from build123d import *

# Parameters (mm, degrees)
EXTRUDE_1_DEPTH             = 90
SKETCH_2_W                  = 90
SKETCH_2_H                  = 44.25
EXTRUDE_2_DEPTH             = 8.2
SKETCH_3_W                  = 90
SKETCH_3_H                  = 102.45
EXTRUDE_3_DEPTH             = 8.2
SKETCH_4_W                  = 4.5
SKETCH_4_H                  = 3.95
CUT_EXTRUDE_1_DEPTH         = 91
SKETCH_5_W                  = 2.25
SKETCH_5_H                  = 3.95
CUT_EXTRUDE_2_DEPTH         = 91
SKETCH_6_W                  = 3.95
SKETCH_6_H                  = 2.25
CUT_EXTRUDE_3_DEPTH         = 91
SKETCH_7_W                  = 3.95
SKETCH_7_H                  = 29.5
CUT_EXTRUDE_4_DEPTH         = 91
SKETCH_8_W                  = 3.95
SKETCH_8_H                  = 9
CUT_EXTRUDE_5_DEPTH         = 91
SKETCH_9_W                  = 3.95
SKETCH_9_H                  = 29.5
CUT_EXTRUDE_6_DEPTH         = 91
SKETCH_10_W                 = 3.95
SKETCH_10_H                 = 6.2
CUT_EXTRUDE_7_DEPTH         = 91
SKETCH_11_W                 = 2.25
SKETCH_11_H                 = 3.95
CUT_EXTRUDE_8_DEPTH         = 91
SKETCH_12_W                 = 4.5
SKETCH_12_H                 = 3.95
CUT_EXTRUDE_9_DEPTH         = 91
SKETCH_13_W                 = 9
SKETCH_13_H                 = 3.95
CUT_EXTRUDE_10_DEPTH        = 91
SKETCH_14_W                 = 46.1
SKETCH_14_H                 = 96.1
CUT_EXTRUDE_11_DEPTH        = 86.6
HOLE_WIZARD_2_5_2_5_1_D     = 2.5
HOLE_WIZARD_2_5_2_5_1_DEPTH = 90
HOLE_WIZARD_4_5_4_5_1_D     = 4.5
HOLE_WIZARD_4_5_4_5_1_DEPTH = 90
SKETCH_22_R                 = 1.631577579
SKETCH_22_R_2               = 1.519375383
SKETCH_22_R_3               = 1.487580747
SKETCH_22_R_4               = 1.581735942
SKETCH_22_R_5               = 1.487835557
SKETCH_22_R_6               = 1.42600834
SKETCH_22_R_7               = 1.628129915
SKETCH_22_R_8               = 1.52367125
EXTRUDE_4_DEPTH             = 90
FILLET_5_R                  = 2
FILLET_6_R                  = 2
FILLET_7_R                  = 2
FILLET_8_R                  = 2
FILLET_9_R                  = 2
FILLET_10_R                 = 2
FILLET_11_R                 = 2
FILLET_12_R                 = 2
FILLET_13_R                 = 2
FILLET_14_R                 = 2
FILLET_15_R                 = 2
FILLET_16_R                 = 2
FILLET_17_R                 = 2
FILLET_18_R                 = 2
FILLET_19_R                 = 2
FILLET_20_R                 = 2
EXTRUDE_6_DEPTH             = 0.2


with BuildPart() as part:
    # Эскиз1 → Бобышка-Вытянуть1 (new body)
    with BuildSketch(Plane(origin=(90, 0, 0), x_dir=(0, 0, -1), z_dir=(1, 0, 0))):
        with BuildLine():
            Line((6.75, 225.906238208), (6.75, 320.75))
            Line((6.75, 320.75), (-38.093761792, 320.75))
            ThreePointArc((-38.093761792, 320.75), (-41.825, 319.5), (-38.093761792, 318.25))
            Line((-38.093761792, 318.25), (-37.5, 318.25))
            Line((-37.5, 318.25), (-37.5, 284.75))
            Line((-37.5, 284.75), (-38.093761792, 284.75))
            ThreePointArc((-38.093761792, 284.75), (-41.825, 283.5), (-38.093761792, 282.25))
            Line((-38.093761792, 282.25), (-37.5, 282.25))
            Line((-37.5, 282.25), (-37.5, 269.25))
            Line((-37.5, 269.25), (-38.093761792, 269.25))
            ThreePointArc((-38.093761792, 269.25), (-41.825, 268), (-38.093761792, 266.75))
            Line((-38.093761792, 266.75), (-37.5, 266.75))
            Line((-37.5, 266.75), (-37.5, 233.25))
            Line((-37.5, 233.25), (-38.093761792, 233.25))
            ThreePointArc((-38.093761792, 233.25), (-41.825, 232), (-38.093761792, 230.75))
            Line((-38.093761792, 230.75), (-37.5, 230.75))
            Line((-37.5, 230.75), (-37.5, 226.5))
            Line((-37.5, 226.5), (-33.25, 226.5))
            Line((-33.25, 226.5), (-33.25, 225.906238208))
            ThreePointArc((-33.25, 225.906238208), (-32, 222.175), (-30.75, 225.906238208))
            Line((-30.75, 225.906238208), (-30.75, 226.5))
            Line((-30.75, 226.5), (-22.25, 226.5))
            Line((-22.25, 226.5), (-22.25, 225.906238208))
            ThreePointArc((-22.25, 225.906238208), (-21, 222.175), (-19.75, 225.906238208))
            Line((-19.75, 225.906238208), (-19.75, 226.5))
            Line((-19.75, 226.5), (-6.75, 226.5))
            Line((-6.75, 226.5), (-6.75, 225.906238208))
            ThreePointArc((-6.75, 225.906238208), (-5.5, 222.175), (-4.25, 225.906238208))
            Line((-4.25, 225.906238208), (-4.25, 226.5))
            Line((-4.25, 226.5), (4.25, 226.5))
            Line((4.25, 226.5), (4.25, 225.906238208))
            ThreePointArc((4.25, 225.906238208), (5.5, 222.175), (6.75, 225.906238208))
        make_face()
    extrude(amount=-EXTRUDE_1_DEPTH)

    # Эскиз2 → Бобышка-Вытянуть2 (add)
    with BuildSketch(Plane(origin=(0, 320.75, 0), x_dir=(-1, 0, 0), z_dir=(0, 1, 0))):
        with Locations((-45, 15.375)):
            Rectangle(SKETCH_2_W, SKETCH_2_H)
    extrude(amount=EXTRUDE_2_DEPTH)

    # Эскиз3 → Бобышка-Вытянуть3 (add)
    with BuildSketch(Plane(origin=(0, 0, -6.75), x_dir=(-1, 0, 0), z_dir=(0, 0, -1))):
        with Locations((-45, 277.725)):
            Rectangle(SKETCH_3_W, SKETCH_3_H)
    extrude(amount=EXTRUDE_3_DEPTH)

    # Эскиз4 → Вырез-Вытянуть1 (cut, through all)
    with BuildSketch(Plane.ZY):
        with Locations((26.5, 326.975)):
            Rectangle(SKETCH_4_W, SKETCH_4_H)
    extrude(amount=-CUT_EXTRUDE_1_DEPTH, mode=Mode.SUBTRACT)

    # Эскиз5 → Вырез-Вытянуть2 (cut, through all)
    with BuildSketch(Plane.ZY):
        with Locations((36.375, 326.975)):
            Rectangle(SKETCH_5_W, SKETCH_5_H)
    extrude(amount=-CUT_EXTRUDE_2_DEPTH, mode=Mode.SUBTRACT)

    # Эскиз6 → Вырез-Вытянуть3 (cut, through all)
    with BuildSketch(Plane.ZY):
        with Locations((-12.975, 227.625)):
            Rectangle(SKETCH_6_W, SKETCH_6_H)
    extrude(amount=-CUT_EXTRUDE_3_DEPTH, mode=Mode.SUBTRACT)

    # Эскиз7 → Вырез-Вытянуть4 (cut, through all)
    with BuildSketch(Plane.ZY):
        with Locations((-12.975, 250)):
            Rectangle(SKETCH_7_W, SKETCH_7_H)
    extrude(amount=-CUT_EXTRUDE_4_DEPTH, mode=Mode.SUBTRACT)

    # Эскиз8 → Вырез-Вытянуть5 (cut, through all)
    with BuildSketch(Plane.ZY):
        with Locations((-12.975, 275.75)):
            Rectangle(SKETCH_8_W, SKETCH_8_H)
    extrude(amount=-CUT_EXTRUDE_5_DEPTH, mode=Mode.SUBTRACT)

    # Эскиз9 → Вырез-Вытянуть6 (cut, through all)
    with BuildSketch(Plane.ZY):
        with Locations((-12.975, 301.5)):
            Rectangle(SKETCH_9_W, SKETCH_9_H)
    extrude(amount=-CUT_EXTRUDE_6_DEPTH, mode=Mode.SUBTRACT)

    # Эскиз10 → Вырез-Вытянуть7 (cut, through all)
    with BuildSketch(Plane.ZY):
        with Locations((-12.975, 325.85)):
            Rectangle(SKETCH_10_W, SKETCH_10_H)
    extrude(amount=-CUT_EXTRUDE_7_DEPTH, mode=Mode.SUBTRACT)

    # Эскиз11 → Вырез-Вытянуть8 (cut, through all)
    with BuildSketch(Plane.ZY):
        with Locations((-9.875, 326.975)):
            Rectangle(SKETCH_11_W, SKETCH_11_H)
    extrude(amount=-CUT_EXTRUDE_8_DEPTH, mode=Mode.SUBTRACT)

    # Эскиз12 → Вырез-Вытянуть9 (cut, through all)
    with BuildSketch(Plane.ZY):
        with Locations((0, 326.975)):
            Rectangle(SKETCH_12_W, SKETCH_12_H)
    extrude(amount=-CUT_EXTRUDE_9_DEPTH, mode=Mode.SUBTRACT)

    # Эскиз13 → Вырез-Вытянуть10 (cut, through all)
    with BuildSketch(Plane.ZY):
        with Locations((13.25, 326.975)):
            Rectangle(SKETCH_13_W, SKETCH_13_H)
    extrude(amount=-CUT_EXTRUDE_10_DEPTH, mode=Mode.SUBTRACT)

    # Эскиз14 → Вырез-Вытянуть11 (cut)
    with BuildSketch(Plane(origin=(90, 0, 0), x_dir=(0, 0, -1), z_dir=(1, 0, 0))):
        with Locations((-13.25, 275.75)):
            Rectangle(SKETCH_14_W, SKETCH_14_H)
    extrude(amount=-CUT_EXTRUDE_11_DEPTH, mode=Mode.SUBTRACT)

    # Диаметр отверстия Ø2.5 (2.5)1
    with Locations(Plane(origin=(90, 0, 0), x_dir=(0, 0, -1), z_dir=(1, 0, 0))):
        with Locations((-39.75, 232), (-21, 224.25), (-39.75, 283.5), (-5.5, 224.25), (5.5, 224.25), (-39.75, 319.5), (-39.75, 268), (-32, 224.25)):
            Hole(HOLE_WIZARD_2_5_2_5_1_D / 2, depth=HOLE_WIZARD_2_5_2_5_1_DEPTH)

    # Диаметр отверстия Ø4.5 (4.5)1
    with Locations(Plane.ZY):
        with Locations((21, 327.25), (32, 327.25), (-13.25, 232), (-13.25, 268), (-13.25, 283.5), (-13.25, 319.5), (-5.5, 327.25), (5.5, 327.25)):
            Hole(HOLE_WIZARD_4_5_4_5_1_D / 2, depth=HOLE_WIZARD_4_5_4_5_1_DEPTH)

    # Эскиз22 → Бобышка-Вытянуть4 (add)
    with BuildSketch(Plane(origin=(90, 0, 0), x_dir=(0, 0, -1), z_dir=(1, 0, 0))):
        with Locations((-39.75, 319.5)):
            Circle(SKETCH_22_R)
        with Locations((-39.75, 283.5)):
            Circle(SKETCH_22_R_2)
        with Locations((-39.75, 268)):
            Circle(SKETCH_22_R_3)
        with Locations((-39.75, 232)):
            Circle(SKETCH_22_R_4)
        with Locations((-32, 224.25)):
            Circle(SKETCH_22_R_5)
        with Locations((-21, 224.25)):
            Circle(SKETCH_22_R_6)
        with Locations((-5.5, 224.25)):
            Circle(SKETCH_22_R_7)
        with Locations((5.5, 224.25)):
            Circle(SKETCH_22_R_8)
    extrude(amount=-EXTRUDE_4_DEPTH)

    # Скругление5
    fillet_5_edges = [part.edges().sort_by_distance(p)[0] for p in [
        (45, 325, 35.25),
    ]]
    fillet(fillet_5_edges, radius=FILLET_5_R)

    # Скругление6
    fillet_6_edges = [part.edges().sort_by_distance(p)[0] for p in [
        (45, 325, 28.75),
    ]]
    fillet(fillet_6_edges, radius=FILLET_6_R)

    # Скругление7
    fillet_7_edges = [part.edges().sort_by_distance(p)[0] for p in [
        (45, 325, 24.25),
    ]]
    fillet(fillet_7_edges, radius=FILLET_7_R)

    # Скругление8
    fillet_8_edges = [part.edges().sort_by_distance(p)[0] for p in [
        (45, 325, 17.75),
    ]]
    fillet(fillet_8_edges, radius=FILLET_8_R)

    # Скругление9
    fillet_9_edges = [part.edges().sort_by_distance(p)[0] for p in [
        (45, 325, 8.75),
    ]]
    fillet(fillet_9_edges, radius=FILLET_9_R)

    # Скругление10
    fillet_10_edges = [part.edges().sort_by_distance(p)[0] for p in [
        (45, 325, 2.25),
    ]]
    fillet(fillet_10_edges, radius=FILLET_10_R)

    # Скругление11
    fillet_11_edges = [part.edges().sort_by_distance(p)[0] for p in [
        (45, 325, -2.25),
    ]]
    fillet(fillet_11_edges, radius=FILLET_11_R)

    # Скругление12
    fillet_12_edges = [part.edges().sort_by_distance(p)[0] for p in [
        (45, 325, -8.75),
    ]]
    fillet(fillet_12_edges, radius=FILLET_12_R)

    # Скругление13
    fillet_13_edges = [part.edges().sort_by_distance(p)[0] for p in [
        (45, 322.75, -11),
    ]]
    fillet(fillet_13_edges, radius=FILLET_13_R)

    # Скругление14
    fillet_14_edges = [part.edges().sort_by_distance(p)[0] for p in [
        (45, 316.25, -11),
    ]]
    fillet(fillet_14_edges, radius=FILLET_14_R)

    # Скругление15
    fillet_15_edges = [part.edges().sort_by_distance(p)[0] for p in [
        (45, 286.75, -11),
    ]]
    fillet(fillet_15_edges, radius=FILLET_15_R)

    # Скругление16
    fillet_16_edges = [part.edges().sort_by_distance(p)[0] for p in [
        (45, 280.25, -11),
    ]]
    fillet(fillet_16_edges, radius=FILLET_16_R)

    # Скругление17
    fillet_17_edges = [part.edges().sort_by_distance(p)[0] for p in [
        (45, 271.25, -11),
    ]]
    fillet(fillet_17_edges, radius=FILLET_17_R)

    # Скругление18
    fillet_18_edges = [part.edges().sort_by_distance(p)[0] for p in [
        (45, 264.75, -11),
    ]]
    fillet(fillet_18_edges, radius=FILLET_18_R)

    # Скругление19
    fillet_19_edges = [part.edges().sort_by_distance(p)[0] for p in [
        (45, 235.25, -11),
    ]]
    fillet(fillet_19_edges, radius=FILLET_19_R)

    # Скругление20
    fillet_20_edges = [part.edges().sort_by_distance(p)[0] for p in [
        (45, 228.75, -11),
    ]]
    fillet(fillet_20_edges, radius=FILLET_20_R)

    # Эскиз23 → Бобышка-Вытянуть6 (add)
    with BuildSketch(Plane.ZY):
        with BuildLine():
            Line((-14.95, 316.81563549), (-3.138029851, 328.95))
            ThreePointArc((-3.138029851, 328.95), (-18.81411193, 332.393335916), (-14.95, 316.81563549))
        make_face()
        with BuildLine():
            Line((41.825, 319.5), (29.638029851, 328.95))
            ThreePointArc((29.638029851, 328.95), (43.851377387, 334.69658957), (41.825, 319.5))
        make_face()
        with BuildLine():
            Line((-14.95, 234.361970149), (-5.5, 222.175))
            ThreePointArc((-5.5, 222.175), (-19.166722881, 221.33490928), (-14.95, 234.361970149))
        make_face()
        with BuildLine():
            Line((32, 222.175), (41.825, 232))
            ThreePointArc((41.825, 232), (43.643106303, 220.356893697), (32, 222.175))
        make_face()
    extrude(amount=-EXTRUDE_6_DEPTH)


solid = part.part
The model under review builds one solid part; all positions refer to its coordinate system, in mm. A direction names the side the tool comes from. Give positions to 0.01 mm unless a question says otherwise; leave off trailing zeros. Order: outer loops, then holes, each group sorted by start corner. A loop starts at its lowest first (then second) coordinate and runs counter-clockwise, first axis right, second up. Notation, with made-up numbers: (78, -32.75) -> (107, -32.75) arc R20 cw to (107, 4.25) -> close; hole circle Ø6 at (-13.5, 39.25). An arc over 180 degrees is marked (long way). Write item = value, one per line. Start each with the question number.
(1) For pin 1 Ø4.5 at (x, y) = (23.5, 228.5) entering from +Z; pin 2 Ø4 at (x, y) = (20.5, 286.5) entering from -Z; pin 3 Ø19 at (y, z) = (324.5, 42) entering from +X; pin 4 Ø2 at (x, z) = (73, -9.5) entering from -Y, all flat-tipped, find the tip position at first contact; note any pin that passes through.
(2) Draft analysis for pull direction Z (two halves, no side actions). For faces 1 (the flat face through (90, 271, 37)), 2 (the cylindrical face through (45.63, 222.176, 21.072)), 3 (the flat face through (44, 301, -11)), state which applies: +Z half, -Z half, draft (parallel to the pull), parting line (faces both ways), or undercut.
(3) For L1, parallel to Y at x = 56.5, z = 32 (3 decimals); L2, parallel to Y at x = 32, z = 23.5; L3, parallel to Z at x = 39, y = 308, list the stretches that pass through material, from the lowest coordinate up. Write a range as from..to.
(4) Take a section at A-A (y = 296.5). Write out the cut boundary in (x, z).
(5) Tool access review of faces 4 (the flat face through (3.4, 276, 14)), 5 (the flat face through (46, 226.5, 27)): name each direction out of +Z, -Z, +X, -X, +Y, -Y from which nothing blocks a thin tool from reaching the whole face with its end or side.
Returned:
q1.pin_1 = 41.41
q1.pin_2 = -14.95
q1.pin_3 = 90
q1.pin_4 = 226.5
q2.face_1 = draft
q2.face_2 = undercut
q2.face_3 = -Z half
q3.L1 = 222.175..227.7, 323.8..325
q3.L2 = 226.5..227.7, 323.8..328.95
q3.L3 = -11..-9.8, 36.3..37.5
q4.outline = (0, -11) -> (90, -11) -> (90, -9.8) -> (3.4, -9.8) -> (3.4, 36.3) -> (90, 36.3) -> (90, 37.5) -> (0, 37.5) -> close
q5.face_4 = +X
q5.face_5 = +X, -X
